Autodesk Inventor part; units mm, degrees
ref_plane "YZ Plane" through (0, 0, 0) normal (1, 0, 0) x (0, 1, 0)
ref_plane "XZ Plane" through (0, 0, 0) normal (0, 1, 0) x (-1, 0, 0)
ref_plane "XY Plane" through (0, 0, 0) normal (0, 0, 1) x (1, 0, 0)
sketch "Sketch5" plane through (0, 0, 0) normal (0, 0, 1) x (1, 0, 0)
  circle A0 centre (0, 0) radius 14.35
  circle A1 centre (0, 0) radius 17.15
  line L0 (32.5, 32.5) -> (-32.5, 32.5)
  line L1 (-32.5, 32.5) -> (-32.5, -32.5)
  line L2 (-32.5, -32.5) -> (32.5, -32.5)
  line L3 (32.5, -32.5) -> (32.5, 32.5)
  line L4 (-27.5, 27.5) -> (27.5, 27.5)
  line L5 (27.5, 27.5) -> (27.5, -27.5)
  line L6 (27.5, -27.5) -> (-27.5, -27.5)
  line L7 (-27.5, -27.5) -> (-27.5, 27.5)
  dimension "d36" = 28.7
  dimension "d37" = 34.3
  dimension "d38" = 65
  dimension "d39" = 65
  dimension "d40" = 55
  dimension "d41" = 55
extrude "Extrusion7" add sketch "Sketch5" along normal blind 10 contours A0 | A1 | L3 L2 L1 L0 | L4 L5 L6 L7
sketch "Sketch6" plane through (0, 0, 0) normal (0, 0, -1) x (-1, 0, 0)
  circle A0 centre (0, 0) radius 14.35
  circle A1 centre (0, 0) radius 17.15
  line L0 (-27.5, 27.5) -> (27.5, 27.5)
  line L1 (27.5, 27.5) -> (27.5, -27.5)
  line L2 (27.5, -27.5) -> (-27.5, -27.5)
  line L3 (-27.5, -27.5) -> (-27.5, 27.5)
  dimension "d44" = 28.7
  dimension "d45" = 34.3
  dimension "d46" = 55
  dimension "d47" = 55
extrude "Extrusion8" cut sketch "Sketch6" against normal blind 5 contours A1
sketch "Sketch7" plane through (0, 0, 10) normal (0, 0, 1) x (1, 0, 0)
  line L0 (-27.5, 27.5) -> (27.5, 27.5)
  line L1 (27.5, 27.5) -> (27.5, -27.5)
  line L2 (27.5, -27.5) -> (-27.5, -27.5)
  line L3 (-27.5, -27.5) -> (-27.5, 27.5)
  point P0 (0, 0)
  dimension "d50" = 55
  dimension "d51" = 55
extrude "Extrusion9" cut sketch "Sketch7" against normal blind 2
properties part number "Clip_MarkerHolderV1"
The model under review builds one solid part; all positions refer to its coordinate system, in mm. A direction names the side the tool comes from. Give positions to 0.01 mm unless a question says otherwise; leave off trailing zeros. Loops run counter-clockwise (first coordinate to the right, second up) from the corner with the lowest first, then second, coordinate; pieces in that order, holes last. Notation, with made-up numbers: (20.25, -11) -> (26.25, -11) arc R18 cw to (26.25, 3) -> close; hole circle Ø1 at (9.25, -27). An arc over 180 degrees is marked (long way). Answer as a JSON object with one key per item and string values. Group by question number.
Q1. Draft analysis for pull direction Y (two halves, no side actions). For faces 4 (the flat face through (0, 32.5, 5)), 5 (the flat face through (4, -14, 5)), 6 (the flat face through (32.5, 0, 5)), state which applies: pulls with the +Y half, pulls with the -Y half, needs draft (parallel to the pull), parting line crosses it, or undercut.
Q2. Take a section at C-C (x = -22.5). Write out the cut boundary in (y, z), plus the area to 3 significant figures.
Q3. Take a section at A-A (x = 0). Write out the cut boundary in (y, z), plus the area to 3 significant figures.
Q4. Take a section at B-B (y = 12). Write out the cut boundary in (x, z).
Q5. Tool access review of faces 1 (the flat face through (-27.5, 0, 9)), 2 (the flat face through (0, -32.5, 5)), 3 (the cylindrical face through (-7.714, 12.1, 2.465)): name each direction out of +Z, -Z, +X, -X, +Y, -Y from which nothing blocks a thin tool from reaching the whole face with its end or side.
Q6. Wall thickness on line 1 along Y through (x, z) = (0, 3.8); line 2 along X through (y, z) = (-12, 9.75); line 3 along X through (y, z) = (-3, 4): over which ranges is each line inside the solid? List them lowest first.
Answer below:
{
 "1": {"face 4": "pulls with the +Y half", "face 5": "undercut", "face 6": "needs draft"},
 "2": {"outline": "(-32.5, 0) -> (32.5, 0) -> (32.5, 10) -> (27.5, 10) -> (27.5, 8) -> (-27.5, 8) -> (-27.5, 10) -> (-32.5, 10) -> close", "area": "540 mm2"},
 "3": {"outline": "(-32.5, 0) -> (-17.15, 0) -> (-17.15, 5) -> (-14.35, 5) -> (-14.35, 0) -> (14.35, 0) -> (14.35, 5) -> (17.15, 5) -> (17.15, 0) -> (32.5, 0) -> (32.5, 10) -> (27.5, 10) -> (27.5, 8) -> (-27.5, 8) -> (-27.5, 10) -> (-32.5, 10) -> close", "area": "512 mm2"},
 "4": {"outline": "(-32.5, 0) -> (-12.25, 0) -> (-12.25, 5) -> (-7.87, 5) -> (-7.87, 0) -> (7.87, 0) -> (7.87, 5) -> (12.25, 5) -> (12.25, 0) -> (32.5, 0) -> (32.5, 10) -> (27.5, 10) -> (27.5, 8) -> (-27.5, 8) -> (-27.5, 10) -> (-32.5, 10) -> close"},
 "5": {"face 1": "+Z", "face 2": "+Z, -Z, +X, -X, -Y", "face 3": "-Z"},
 "6": {"line 1": "y = -32.5 to -17.15, -14.35 to 14.35, 17.15 to 32.5", "line 2": "x = -32.5 to -27.5, 27.5 to 32.5", "line 3": "x = -32.5 to -16.89, -14.03 to 14.03, 16.89 to 32.5"}
}
